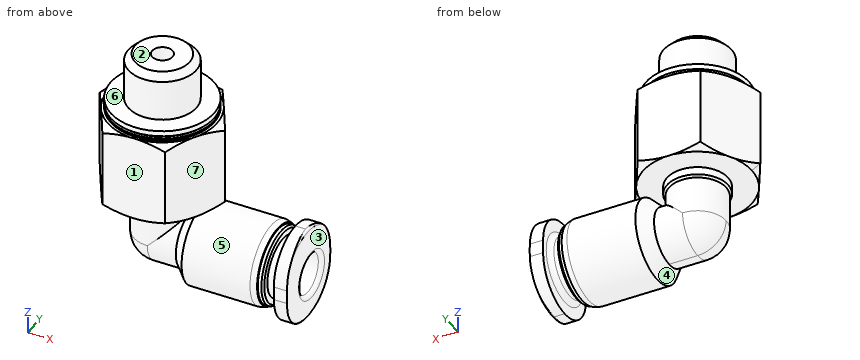
```python
from build123d import *
from build123d.topology import SkipClean

# Parameters (mm, degrees)
LINEAR_AUSTRAGEN1_DEPTH = 1.2
SKIZZE6_W               = 14
SKIZZE6_H               = 0.75
SKIZZE7_W               = 16
SKIZZE7_H               = 16
LINEAR_AUSTRAGEN2_DEPTH = 7.166666667


with BuildPart() as part:
    # Skizze1 → Rotation1 (revolve)
    with BuildSketch(Plane.XY, mode=Mode.PRIVATE) as rotation1_sk:
        with BuildLine():
            Line((0, 2.1), (2.1, 2.1))
            Line((2.1, 2.1), (3, 3))
            Line((3, 3), (8.042857143, 3))
            Line((8.042857143, 3), (8.5, 2.877508941))
            Line((8.5, 2.877508941), (8.5, 2.770329264))
            Line((8.5, 2.770329264), (8.758578644, 2.770329264))
            Line((8.758578644, 2.770329264), (8.9, 2.628907907))
            Line((8.9, 2.628907907), (8.9, 2.2))
            Line((8.9, 2.2), (9.43, 2.2))
            ThreePointArc((9.43, 2.2), (9.691629509, 2.308370491), (9.8, 2.57))
            Line((9.8, 2.57), (9.8, 3.5))
            Line((9.8, 3.5), (10.532424207, 3.5))
            ThreePointArc((10.532424207, 3.5), (10.660981728, 3.453208889), (10.729385757, 3.334729636))
            Line((10.729385757, 3.334729636), (11, 1.8))
            Line((11, 1.8), (11, 0))
            Line((11, 0), (-2.1, 0))
            ThreePointArc((-2.1, 0), (-1.48492424, 1.48492424), (0, 2.1))
        make_face()
    revolve(rotation1_sk.sketch.rotate(Axis((11, 0, 0), (-1, 0, 0)), 90), axis=Axis((11, 0, 0), (-1, 0, 0)))

    # Skizze2 → Rotation2 (revolve)
    with SkipClean():  # the faces are left unmerged after this step: merging them gives an invalid solid
        with BuildSketch(Plane(origin=(0, 0, 0), x_dir=(0, 0, -1), z_dir=(1, 0, 0)), mode=Mode.PRIVATE) as rotation2_sk:
            Polygon((-10.5, 0), (-10.5, 3.8), (-10.1, 3.8), (-10, 3.7), (-9.9, 3.8), (-9.75, 3.8), (-9.75, 4), (-9.380495828, 4.64), (-3.744504172, 4.64), (-3.375, 4), (-3.375, 2.25), (-2.8, 2.25), (-2.65, 2.1), (0, 2.1), (0, 0), align=None)
        revolve(rotation2_sk.sketch.rotate(Axis((0, 0, 0), (0, 0, 1)), 90), axis=Axis((0, 0, 0), (0, 0, 1)))

    # Skizze3 → Rotation3 (revolve)
    with SkipClean():  # the faces are left unmerged after this step: merging them gives an invalid solid
        with BuildSketch(Plane(origin=(0, 0, 0), x_dir=(0, 0, -1), z_dir=(1, 0, 0)), mode=Mode.PRIVATE) as rotation3_sk:
            Polygon((-14, 0), (-14, 2.0095), (-13.5095, 2.5), (-10.5, 2.5), (-10.5, 0), align=None)
        revolve(rotation3_sk.sketch.rotate(Axis((0, 0, 10.5), (0, 0, 1)), 90), axis=Axis((0, 0, 10.5), (0, 0, 1)))

    # Skizze4 → Linear austragen1 (cut)
    with SkipClean():  # the faces are left unmerged after this step: merging them gives an invalid solid
        with BuildSketch(Plane(origin=(11, 0, 0), x_dir=(0, 0, -1), z_dir=(1, 0, 0))):
            Polygon((-4.2, 2.424871131), (-4.2, -2.424871131), (0, -4.849742261), (4.2, -2.424871131), (4.2, 2.424871131), (0, 4.849742261), align=None)
            with BuildLine():
                Line((-0.5, -3), (0.5, -3))
                ThreePointArc((0.5, -3), (2.621320344, -2.121320344), (3.5, 0))
                ThreePointArc((3.5, 0), (2.621320344, 2.121320344), (0.5, 3))
                Line((0.5, 3), (-0.5, 3))
                ThreePointArc((-0.5, 3), (-2.621320344, 2.121320344), (-3.5, 0))
                ThreePointArc((-3.5, 0), (-2.621320344, -2.121320344), (-0.5, -3))
            make_face(mode=Mode.SUBTRACT)
        extrude(amount=-LINEAR_AUSTRAGEN1_DEPTH, mode=Mode.SUBTRACT)

    # Skizze6 → Schnitt-Rotation1 (revolve, cut)
    with SkipClean():  # the faces are left unmerged after this step: merging them gives an invalid solid
        with BuildSketch(Plane(origin=(0, 0, 0), x_dir=(0, 0, -1), z_dir=(1, 0, 0)), mode=Mode.PRIVATE) as schnitt_rotation1_sk:
            with Locations((-7, 0.375)):
                Rectangle(SKIZZE6_W, SKIZZE6_H)
        revolve(schnitt_rotation1_sk.sketch.rotate(Axis((0, 0, 0), (0, 0, 1)), 90), axis=Axis((0, 0, 0), (0, 0, 1)), mode=Mode.SUBTRACT)

    # Skizze5 → Schnitt-Rotation2 (revolve, cut)
    with SkipClean():  # the faces are left unmerged after this step: merging them gives an invalid solid
        with BuildSketch(Plane(origin=(0, 0, 0), x_dir=(1, 0, 0), z_dir=(0, 1, 0))):
            with BuildLine():
                Line((0, 0.75), (1.5, 0.75))
                Line((1.5, 0.75), (1.5, 1.5))
                Line((1.5, 1.5), (10.7, 1.5))
                ThreePointArc((10.7, 1.5), (10.912132034, 1.587867966), (11, 1.8))
                Line((11, 1.8), (11, 0))
                Line((11, 0), (-0.75, 0))
                ThreePointArc((-0.75, 0), (-0.530330086, 0.530330086), (0, 0.75))
            make_face()
        revolve(axis=Axis((11, 0, 0), (-1, 0, 0)), mode=Mode.SUBTRACT)

    # Skizze7 → Linear austragen2 (cut)
    with SkipClean():  # the faces are left unmerged after this step: merging them gives an invalid solid
        with BuildSketch(Plane.XY.offset(10.5)):
            Rectangle(SKIZZE7_W, SKIZZE7_H)
            Polygon((-4.618802154, 0), (-2.309401077, -4), (2.309401077, -4), (4.618802154, 0), (2.309401077, 4), (-2.309401077, 4), align=None, mode=Mode.SUBTRACT)
        extrude(amount=-LINEAR_AUSTRAGEN2_DEPTH, mode=Mode.SUBTRACT)


solid = part.part
```
Part model, mm, in its own coordinate system. Face numbers are marked on the shaded views. A direction names the side the tool comes from. Round coordinates to 2 decimals unless told otherwise and drop trailing zeros. Write each loop counter-clockwise with the first axis right and the second up, starting at its lowest first coordinate (ties: lowest second). Pieces come first, ordered by that corner, then holes. Notation, with made-up numbers: M 24.5,-16 L 82.5,-16 A6 ccw 82.5,-11 Z; hole C 41.25,29.25 d2. An arc over 180 degrees is marked long. Answer as CSV lines item,"result". Start each with the question number.
1) Which spindle directions (+Z, -Z, +X, -X, +Y, -Y) get a long thin tool onto all of the face, cutting with end or side? Do the marked faces 5, 6 and 7. Say none if no direction does.
2) Drop flat-ended pins along their axis: pin 1 (0.5 mm diameter, centred on x = 10, z = 0, fed in from +Y); pin 2 (1.8 mm diameter, centred on y = 0, z = 0, fed in from -X); pin 3 (1.4 mm diameter, centred on x = 0, y = 0, fed in from -Z). Give the stop position or say it passes through.
3) Band-saw the part on A-A (z = 11). List the corners of the cut face in (x, y), then the cut area to 3 significant figures.
4) Mould opens along Z. For the marked faces 1, 2, 3 and 4 say: +Z half, -Z half, draft (parallel to the pull), parting line (faces both ways), or undercut.
5) Drill centre lines: L1, parallel to Y at x = 0.6, z = 0; L2, parallel to Y at x = 5.5, z = 0; L3, parallel to Y at x = -3.75, z = 7. Where is each one in solid material? Low to high.
Worked out:
1,face 5,"none"
1,face 6,"+Z"
1,face 7,"+Z, +X, -Y"
2,pin 1,"y = 3"
2,pin 2,"x = -2.1"
2,pin 3,"z = -2.1"
3,outline,"C 0,0 d5; hole C 0,0 d1.5"
3,area,"17.9 mm²"
4,face 1,"draft"
4,face 2,"+Z half"
4,face 3,"parting line"
4,face 4,"undercut"
5,L1,"-2.1 to -0.75, 0.75 to 2.1"
5,L2,"-3 to -1.5, 1.5 to 3"
5,L3,"-1.5 to 1.5"
